Autodesk Inventor part; units mm, degrees
ref_plane "YZ Plane" through (0, 0, 0) normal (1, 0, 0) x (0, 1, 0)
ref_plane "XZ Plane" through (0, 0, 0) normal (0, 1, 0) x (-1, 0, 0)
ref_plane "XY Plane" through (0, 0, 0) normal (0, 0, 1) x (1, 0, 0)
sketch "Sketch1" plane through (0, 0, 0) normal (0, 1, 0) x (-1, 0, 0)
  line L0 (40, -40) -> (-40, -40)
  line L1 (-40, -40) -> (-40, 40)
  line L2 (-40, 40) -> (40, 40)
  line L3 (40, 40) -> (40, -40)
  line L4 (40, -40) -> (-40, 40) construction
  line L5 (-40, -40) -> (40, 40) construction
  line L6 (-37, -37) -> (37, -37)
  line L7 (37, -37) -> (37, 37)
  line L8 (37, 37) -> (-37, 37)
  line L9 (-37, 37) -> (-37, -37)
  point P0 (0, 0)
  dimension "d0" = 3
  dimension "d1" = 80
extrude "Extrusion1" add sketch "Sketch1" along normal blind 374.705
sketch "Sketch2" plane through (0, 0, 0) normal (1, 0, 0) x (0, 1, 0)
  line L0 (0, 40) -> (0, -40) construction
  line L1 (0, -40) -> (374.705, -40)
  line L2 (374.705, 40) -> (374.705, -40)
  line L3 (0, 40) -> (374.705, 40)
  line L4 (0, -40) -> (374.705, -40)
  line L5 (374.705, -40) -> (342.6109, 40)
  point P0 (0, 0)
  dimension "d4" = 21.86
extrude "Extrusion2" cut sketch "Sketch2" along normal through all both and the other way through all
equation "\"d1\" = Legs_Tube_dim"
equation "\"d4\" = Legs_Tube_cut_angle"
properties part number "PRS 9681 leg tube_D1200 940"
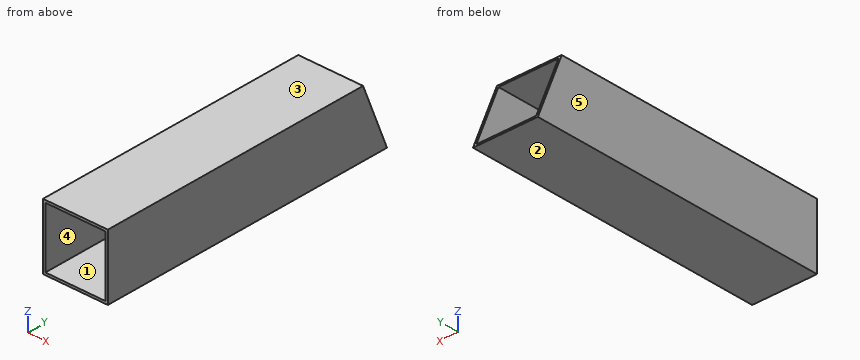
Source: CAD feature listing. Evaluate the final solid. Frame: model axes, mm. Face numbers are marked on the shaded views. A direction names the side the tool comes from. Give positions to 0.01 mm unless a question says otherwise; leave off trailing zeros. Loops run counter-clockwise (first coordinate to the right, second up) from the corner with the lowest first, then second, coordinate; pieces in that order, holes last. Notation, with made-up numbers: (-27, -11.75) -> (19, -11.75) arc R21 cw to (19, 2.25) -> close; hole circle Ø7 at (53, 67). An arc over 180 degrees is marked (long way). Use a Markdown table: item, result. Add a question column.
(1) Section query A-A (x = -8). Output: boundary loops of the cut face in (y, z) (3 decimals), then the cut area to 3 significant figures.
(2) Access query for the marked faces 1 and 2. Directions: +Z, -Z, +X, -X, +Y, -Y. A direction counts if a zero-diameter tool reaches every point of the face in a straight line with its end or side. Return the directions, or none.
(3) Section query C-C (y = 108.5). Output: boundary loops of the cut face in (x, z), then the cut area to 3 significant figures.
(4) Pull-direction query (X, two-part tool) for the marked faces 3, 4 and 5; classes: +X half, -X half, draft (parallel to the pull), parting line (faces both ways), or undercut.
(5) Section query B-B (z = -14). Output: boundary loops of the cut face in (x, y), then the cut area to 3 significant figures.
(6) Ray query, line 1 (X direction, y = 52, z = -19.5). Return the intervals inside material, ascending.
Checked values:
| question | item | result |
|---|---|---|
| 1 | outline | (0, -40) -> (374.705, -40) -> (373.501, -37) -> (0, -37) -> close; (0, 37) -> (343.814, 37) -> (342.611, 40) -> (0, 40) -> close |
| 1 | area | 2,150 mm^2 |
| 2 | face 1 | +Y, -Y |
| 2 | face 2 | -Z, +X, -X, +Y, -Y |
| 3 | outline | (-40, -40) -> (40, -40) -> (40, 40) -> (-40, 40) -> close; hole (-37, -37) -> (37, -37) -> (37, 37) -> (-37, 37) -> close |
| 3 | area | 924 mm^2 |
| 4 | face 3 | draft |
| 4 | face 4 | undercut |
| 4 | face 5 | -X half |
| 5 | outline | (-40, 0) -> (-37, 0) -> (-37, 364.27) -> (-40, 364.27) -> close; (37, 0) -> (40, 0) -> (40, 364.27) -> (37, 364.27) -> close |
| 5 | area | 2,190 mm^2 |
| 6 | line 1 | -40 to -37, 37 to 40 |
